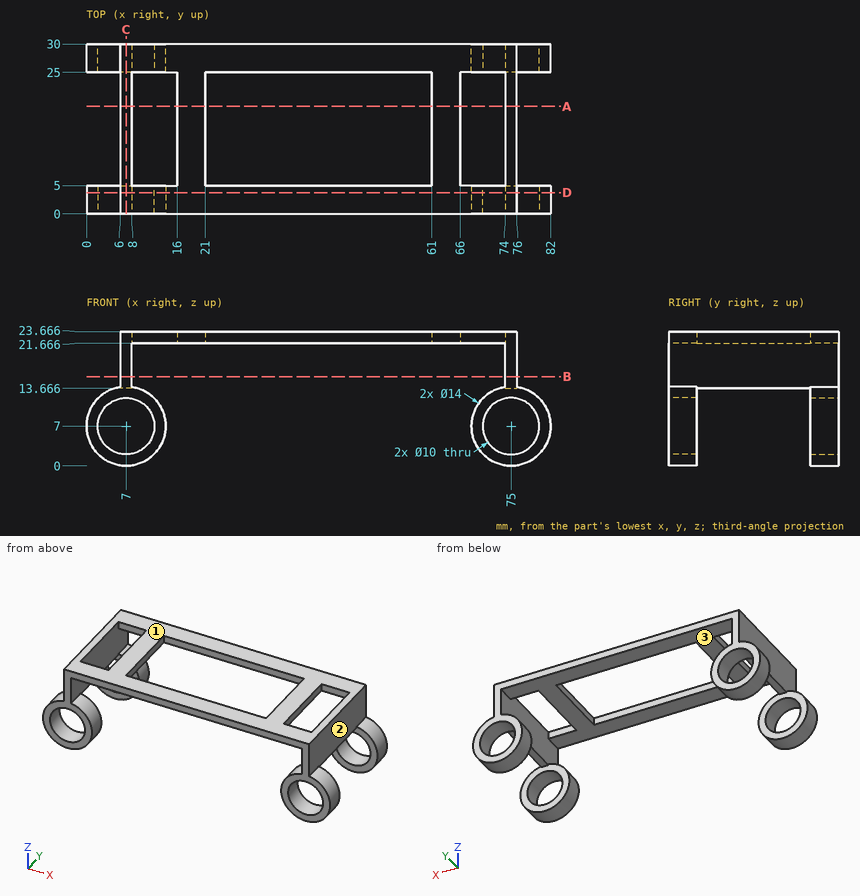
Geometry check sheet. Reference: drawing and pictorial views, mm from the part's lowest x, y, z. Give positions to 0.01 mm unless a question says otherwise; leave off trailing zeros. Order: outer loops, then holes, each group sorted by start corner. A loop starts at its lowest first (then second) coordinate and runs counter-clockwise, first axis right, second up. Notation, with made-up numbers: (5.25, 8.25) -> (38.25, 8.25) arc R12 cw to (38.25, 22.25) -> close; hole circle Ø4 at (29.25, 10). An arc over 180 degrees is marked (long way). Write each question's results on one line, items separated by ' | '. Start each with the question number.
(1) Scan lines: line 1 (X direction, y = 2.6, z = 7); line 2 (X direction, y = 25.25, z = 18); line 3 (Z direction, x = 75, y = 1.65). Record each from-to range of solid material in increasing order.
(2) Sectioned sample at D-D (y = 3.75). Enter the section's corners in (x, z).
(3) Sectioned sample at B-B (z = 15.75). Enter the section's corners in (x, y), plus the area to 3 significant figures.
(4) Sectioned sample at A-A (y = 19). Enter the section's corners in (x, z), plus the area to 3 significant figures.
(5) Sectioned sample at C-C (x = 7). Enter the section's corners in (y, z).
(6) Mould release check, pull along Z, two halves, no side actions. Record for the marked faces 1, 2 and 3: pulls with the +Z half, pulls with the -Z half, needs draft (parallel to the pull), parting line crosses it, or undercut.
(7) Gauge pin test, flat ends, axial feed: P1, Ø6, axis at x = 75, z = 7, coming from the +Y side (3 decimals); P2, Ø4, axis at y = 15, z = 16, coming from the +X side; P3, Ø1.6, axis at y = 18.5, z = 22.5, coming from the -X side. Record the tip position at first contact, or that the pin passes through.
Answer below:
1) line 1: 0 to 2, 12 to 14, 68 to 70, 80 to 82 | line 2: 6 to 8, 74 to 76 | line 3: 0 to 2, 12 to 23.67
2) outline: (6, 13.93) arc R7 ccw (long way) to (8, 13.93) -> (8, 21.67) -> (74, 21.67) -> (74, 13.93) arc R7 ccw (long way) to (76, 13.93) -> (76, 23.67) -> (6, 23.67) -> close; hole circle Ø10 at (7, 7); hole circle Ø10 at (75, 7)
3) outline: (6, 0) -> (8, 0) -> (8, 30) -> (6, 30) -> close; (74, 0) -> (76, 0) -> (76, 30) -> (74, 30) -> close | area: 120 mm2
4) outline: (6, 13.67) -> (8, 13.67) -> (8, 23.67) -> (6, 23.67) -> close; (16, 21.67) -> (21, 21.67) -> (21, 23.67) -> (16, 23.67) -> close; (61, 21.67) -> (66, 21.67) -> (66, 23.67) -> (61, 23.67) -> close; (74, 13.67) -> (76, 13.67) -> (76, 23.67) -> (74, 23.67) -> close | area: 60.0 mm2
5) outline: (0, 0) -> (5, 0) -> (5, 2) -> (0, 2) -> close; (0, 12) -> (5, 12) -> (5, 13.67) -> (25, 13.67) -> (25, 12) -> (30, 12) -> (30, 23.67) -> (0, 23.67) -> close; (25, 0) -> (30, 0) -> (30, 2) -> (25, 2) -> close
6) face 1: pulls with the +Z half | face 2: needs draft | face 3: undercut
7) P1: through | P2: x = 76 | P3: x = 6
